Check sheet for the modelled part. Datum: model origin and axes. Units: mm. A direction names the side the tool comes from. Round coordinates to 2 decimals unless told otherwise and drop trailing zeros.
```python
from build123d import *
from OCP.BRepAlgoAPI import BRepAlgoAPI_Cut
from OCP.TopTools import TopTools_ListOfShape

# Parameters (mm, degrees)
BOSS_EXTRUDE8_DEPTH      = 152.4
FILLET4_R                = 25.4
FILLET5_R                = 25.4
FILLET6_R                = 25.4
FILLET7_R                = 25.4
CUT_EXTRUDE16_DEPTH      = 247.514886375
CUT_EXTRUDE16_DEPTH_BACK = 247.514886375
SKETCH15_OUTSIDE_W       = 225.302
SKETCH15_OUTSIDE_H       = 267.354
CUT_EXTRUDE15_START      = -139.7
CUT_EXTRUDE15_DEPTH      = 139.7
CUT_EXTRUDE15_START_2    = -107.121047974
CUT_EXTRUDE15_2_DEPTH    = 215.583659042
FILLET10_R               = 12.7
CUT_EXTRUDE17_DEPTH      = 88.9


with BuildPart() as part:
    # Sketch8 → Boss-Extrude8 (new body)
    with BuildSketch(Plane(origin=(0, 0, 0), x_dir=(0, 0, -1), z_dir=(1, 0, 0))):
        with BuildLine():
            add(Edge.make_bspline(
                [(-89.517321988, -36.735442624), (-0.634104952, -60.975176902), (88.282437318, -37.028001665)],
                knots=[0, 0, 0, 1, 1, 1], degree=2))
            add(Edge.make_bspline(
                [(113.698608464, 137.87777005), (148.206005145, 51.814722278), (88.282437318, -37.028001665)],
                knots=[0, 0, 0, 1, 1, 1], degree=2))
            add(Edge.make_bspline(
                [(-114.901391536, 137.87777005), (-0.596034429, 153.168104446), (113.698608464, 137.87777005)],
                knots=[0, 0, 0, 1, 1, 1], degree=2))
            add(Edge.make_bspline(
                [(-114.901391536, 137.87777005), (-150.307927624, 52.141383045), (-89.517321988, -36.735442624)],
                knots=[0, 0, 0, 1, 1, 1], degree=2))
        make_face()
    extrude(amount=BOSS_EXTRUDE8_DEPTH)

    # Fillet4
    fillet4_edges = [part.edges().sort_by_distance(p)[0] for p in [
        (76.2, 137.87777005, 114.901391536),
    ]]
    fillet(fillet4_edges, radius=FILLET4_R)

    # Fillet5
    fillet5_edges = [part.edges().sort_by_distance(p)[0] for p in [
        (76.2, -36.735442624, 89.517321988),
    ]]
    fillet(fillet5_edges, radius=FILLET5_R)

    # Fillet6
    fillet6_edges = [part.edges().sort_by_distance(p)[0] for p in [
        (76.2, -37.028001665, -88.282437318),
    ]]
    fillet(fillet6_edges, radius=FILLET6_R)

    # Fillet7
    fillet7_edges = [part.edges().sort_by_distance(p)[0] for p in [
        (76.2, 137.87777005, -113.698608464),
    ]]
    fillet(fillet7_edges, radius=FILLET7_R)


with BuildPart() as cut_extrude16_tool:
    # Sketch15 outside → Cut-Extrude16 (new, two sides: drawn at the far end of the back side and taken through both)
    with BuildSketch(Plane.XY.offset(-CUT_EXTRUDE16_DEPTH_BACK)):
        with Locations((76.2, 48.297)):
            Rectangle(SKETCH15_OUTSIDE_W, SKETCH15_OUTSIDE_H)
        with BuildLine():
            Line((0, 145.522937248), (152.4, 145.522937248))
            Line((152.4, 145.522937248), (152.4, -48.92889358))
            add(Edge.make_bspline(
                [(152.4, -48.92889358), (110.926936948, -4.126097701), (19.317462744, -43.320532891), (0, 25.209390068)],
                knots=[0, 0, 0, 0, 1, 1, 1, 1], degree=3))
            Line((0, 25.209390068), (0, 145.522937248))
        make_face(mode=Mode.SUBTRACT)
    extrude(amount=CUT_EXTRUDE16_DEPTH + CUT_EXTRUDE16_DEPTH_BACK)


with BuildPart() as part_1:
    add(part.part)

    # Cut-Extrude16: cut by cut_extrude16_tool, with a tolerance
    cut_extrude16_stock = TopTools_ListOfShape()
    cut_extrude16_stock.Append(part_1.part.wrapped)
    cut_extrude16_tools = TopTools_ListOfShape()
    cut_extrude16_tools.Append(cut_extrude16_tool.part.wrapped)
    cut_extrude16_cut = BRepAlgoAPI_Cut()
    cut_extrude16_cut.SetArguments(cut_extrude16_stock)
    cut_extrude16_cut.SetTools(cut_extrude16_tools)
    cut_extrude16_cut.SetFuzzyValue(0.00001)
    cut_extrude16_cut.Build()
    add(Compound.cast(cut_extrude16_cut.Shape()).solids(), mode=Mode.REPLACE)

    # Cut-Extrude15: read off the stored shape, not the designer's step
    # Cut-Extrude15 outline → Cut-Extrude15 (cut)
    with BuildSketch(Plane(origin=(152.4, 0, 0), x_dir=(0, 0, -1), z_dir=(1, 0, 0)).offset(CUT_EXTRUDE15_START)):
        with BuildLine():
            Line((-108.462610918, 118.343948744), (-108.462610968, 29.857145502))
            add(Edge.make_bspline(
                [(-108.462610968, 29.857145502), (-108.303396792, 29.330392086), (-108.141581561, 28.80417359), (-107.065329269, 25.362622105), (-106.073914967, 22.462725385), (-103.939463928, 16.695703636), (-102.803256247, 13.846836756), (-101.052061435, 9.735706989), (-100.487342065, 8.448198791), (-99.909630865, 7.167215308)],
                knots=[0.613732154, 0.613732154, 0.613732154, 0.613732154, 0.625, 0.625, 0.6875, 0.6875, 0.75, 0.75, 0.77871627, 0.77871627, 0.77871627, 0.77871627], degree=3))
            Line((-99.909630865, 7.167215308), (98.50890353, 7.1672153))
            add(Edge.make_bspline(
                [(98.50890353, 7.1672153), (99.030702422, 8.344757297), (99.541287229, 9.526823546), (102.383358501, 16.284548345), (104.473090717, 21.957741134), (106.563539536, 28.680710786), (106.846143617, 29.616761908), (107.121047874, 30.555919476)],
                knots=[0.223373266, 0.223373266, 0.223373266, 0.223373266, 0.25, 0.25, 0.375, 0.375, 0.395143119, 0.395143119, 0.395143119, 0.395143119], degree=3))
            Line((107.121047874, 30.555919476), (107.121047874, 118.246293452))
            ThreePointArc((107.121047874, 118.246293452), (103.111414114, 124.347995452), (96.404571724, 127.233510198))
            Line((96.404571724, 127.233510198), (-97.784453574, 127.21292508))
            ThreePointArc((-97.784453574, 127.21292508), (-104.442431868, 124.366378649), (-108.462610918, 118.343948744))
        make_face()
    extrude(amount=CUT_EXTRUDE15_DEPTH, mode=Mode.SUBTRACT)

    # Cut-Extrude15 2 outline → Cut-Extrude15 2 (add)
    with BuildSketch(Plane.XY.offset(CUT_EXTRUDE15_START_2)):
        with BuildLine():
            Line((12.7, 7.167215307), (20.89442948, 7.1672153))
            add(Edge.make_bspline(
                [(20.89442948, 7.1672153), (17.477928889, 12.167382595), (14.701088569, 18.110401588), (12.7, 25.209390068)],
                knots=[0.896410383, 0.896410383, 0.896410383, 0.896410383, 1, 1, 1, 1], degree=3))
            Line((12.7, 25.209390068), (12.7, 7.167215307))
        make_face()
    extrude(amount=CUT_EXTRUDE15_2_DEPTH)

    # Fillet10
    fillet10_edges = [part_1.edges().sort_by_distance(p)[0] for p in [
        (0, 25.209390068, 60.161160898),
    ]]
    fillet(fillet10_edges, radius=FILLET10_R)

    # Sketch17 → Cut-Extrude17 (cut)
    with BuildSketch(Plane(origin=(152.4, 0, 0), x_dir=(0, 0, -1), z_dir=(1, 0, 0))):
        Polygon((-99.909630865, 7.167215308), (-79.922490142, -12.819925415), (78.521762811, -12.819925415), (98.508903533, 7.167215308), align=None)
    extrude(amount=-CUT_EXTRUDE17_DEPTH, mode=Mode.SUBTRACT)


solid = part_1.part
```
Item 1: Release check for a two-part mould opening along Z. For faces 3 (the cylindrical face through (81.57, 124.28, -103.19)), 4 (the flat face through (0, 76, 3)) record: released by +Z, released by -Z, zero draft, split by the parting line, or undercut.
Answer:
face 3: undercut
face 4: zero draft
Item 2: Go/stop test with flat-tipped pins: P1, Ø4, axis at x = 79.5, y = 2.5, coming from the +Z side; P2, Ø13, axis at x = 40.5, z = 2, coming from the +Y side; P3, Ø1.5, axis at x = 126, z = -42.5, coming from the +Y side; P4, Ø12, axis at x = 39.5, y = 111.5, coming from the -Z side. Record where each tip stops, or that it passes through.
Answer:
P1: stops at z = 112.62
P2: stops at y = 145.52
P3: stops at y = 144.47
P4: stops at z = -123.32
Item 3: Scan lines: line 1 along Y through (x, z) = (15.5, -41); line 2 along Z through (x, y) = (23, 50); line 3 along Y through (x, z) = (114, -95). Record each from-to range of solid material in increasing order.
Answer:
line 1: y = -1.33 to 17.15, 127.23 to 144.51
line 2: z = -124.43 to -107.12, 108.46 to 126.06
line 3: y = -26.59 to 3.66, 127.23 to 140.17
Item 4: Access from +Z, -Z, +X, -X, +Y, -Y to the whole of each face (thin tool, end or side, straight path). Record for faces 1 (the flat face through (12.7, 77, 2)), 2 (the flat face through (152.4, -15, -9)).
Answer:
face 1: +X
face 2: +Z, -Z, +X, +Y, -Y
